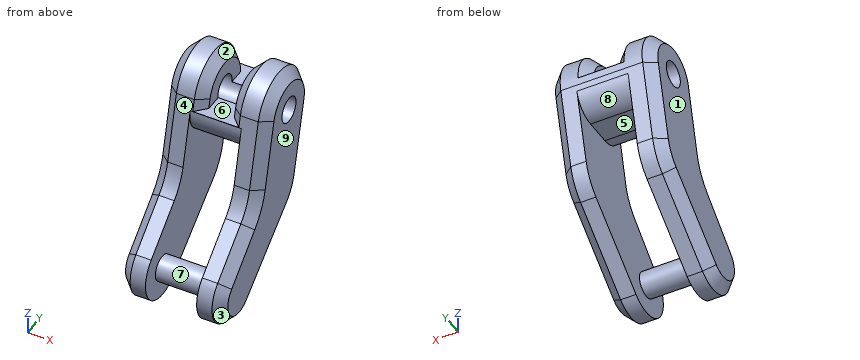
from build123d import *

# Parameters (mm, degrees)
SKETCH1_R               = 2.5
BOSS_EXTRUDE1_DEPTH     = 20
SKETCH2_W               = 10
SKETCH2_H               = 31.25301739
CUT_EXTRUDE1_DEPTH      = 26.258397403
CUT_EXTRUDE1_DEPTH_BACK = 7
FILLET1_R               = 5
CHAMFER1_SIZE           = 2
SKETCH4_R               = 2.5
BOSS_EXTRUDE2_DEPTH     = 20
SKETCH5_W               = 5
SKETCH5_H               = 8
CUT_EXTRUDE2_DEPTH      = 26.258397403
CUT_EXTRUDE2_DEPTH_BACK = 7
CHAMFER2_SIZE           = 2
SCALE1_SCALE            = 2


with BuildPart() as part:
    # Sketch1 → Boss-Extrude1 (new body)
    with BuildSketch(Plane(origin=(0, 0, 0), x_dir=(0, 0, -1), z_dir=(1, 0, 0))):
        with BuildLine():
            Line((-26.320929868, 25.036498407), (-12.043816775, 21.484201108))
            ThreePointArc((-12.043816775, 21.484201108), (-9.046440649, 20.189090541), (-6.626054873, 17.99744556))
            Line((-6.626054873, 17.99744556), (4.699352175, 3.730427474))
            ThreePointArc((4.699352175, 3.730427474), (3.853673118, -4.598826318), (-4.495069155, -3.974211028))
            Line((-4.495069155, -3.974211028), (-11.760416857, 4.243329543))
            ThreePointArc((-11.760416857, 4.243329543), (-14.097354711, 6.188634088), (-16.910883072, 7.341693702))
            Line((-16.910883072, 7.341693702), (-29.887785442, 10.466860499))
            ThreePointArc((-29.887785442, 10.466860499), (-35.416669297, 19.541837843), (-26.320929868, 25.036498407))
        make_face()
        Circle(SKETCH1_R, mode=Mode.SUBTRACT)
        with Locations((-28.13179866, 17.758397403)):
            Circle(SKETCH1_R, mode=Mode.SUBTRACT)
    extrude(amount=BOSS_EXTRUDE1_DEPTH)

    # Sketch2 → Cut-Extrude1 (cut, two sides)
    with BuildSketch(Plane(origin=(0, 0, 0), x_dir=(1, 0, 0), z_dir=(0, 1, 0))) as cut_extrude1_sk:
        with Locations((10, -5.807345092)):
            Rectangle(SKETCH2_W, SKETCH2_H)
    extrude(amount=CUT_EXTRUDE1_DEPTH, mode=Mode.SUBTRACT)
    extrude(cut_extrude1_sk.sketch, amount=-CUT_EXTRUDE1_DEPTH_BACK, mode=Mode.SUBTRACT)

    # Fillet1
    fillet1_edges = [part.edges().sort_by_distance(p)[0] for p in [
        (10, 23.820541998, 21.433853787),
        (10, 8.430939618, 21.433853787),
    ]]
    fillet(fillet1_edges, radius=FILLET1_R)

    # Chamfer1
    chamfer1_edges = [part.edges().sort_by_distance(p)[0] for p in [
        (20, 6.188634088, 14.097354711),
        (0, 8.904277101, 23.399334257),
        (0, 19.541837843, 35.416669297),
        (20, 0.134559258, 8.127743006),
        (20, -4.598826318, -3.853673118),
        (20, 10.863936517, 0.963351349),
        (20, 20.189090541, 9.046440649),
        (20, 23.260349758, 19.182373322),
        (20, 19.541837843, 35.416669297),
        (20, 8.904277101, 23.399334257),
        (0, 23.260349758, 19.182373322),
        (0, 20.189090541, 9.046440649),
        (0, 10.863936517, 0.963351349),
        (0, -4.598826318, -3.853673118),
        (0, 0.134559258, 8.127743006),
        (0, 6.188634088, 14.097354711),
    ]]
    chamfer(chamfer1_edges, length=CHAMFER1_SIZE)

    # Sketch4 → Boss-Extrude2 (add)
    with BuildSketch(Plane(origin=(20, 0, 0), x_dir=(0, 0, -1), z_dir=(1, 0, 0))):
        Circle(SKETCH4_R)
    extrude(amount=-BOSS_EXTRUDE2_DEPTH)

    # Sketch5 → Cut-Extrude2 (cut, two sides)
    with BuildSketch(Plane(origin=(0, 0, 0), x_dir=(1, 0, 0), z_dir=(0, 1, 0))) as cut_extrude2_sk:
        with Locations((10, -31.63179866)):
            Rectangle(SKETCH5_W, SKETCH5_H)
    extrude(amount=CUT_EXTRUDE2_DEPTH, mode=Mode.SUBTRACT)
    extrude(cut_extrude2_sk.sketch, amount=-CUT_EXTRUDE2_DEPTH_BACK, mode=Mode.SUBTRACT)

    # Chamfer2
    chamfer2_edges = [part.edges().sort_by_distance(p)[0] for p in [
        (7.5, 18.890459141, 35.545868812),
        (7.5, 10.195211119, 28.759792051),
        (12.5, 18.890459141, 35.545868812),
        (12.5, 10.195211119, 28.759792051),
    ]]
    chamfer(chamfer2_edges, length=CHAMFER2_SIZE)


with BuildPart() as part_1:
    # Scale1: scaled about (10, 12.009955127, 15.525619082)
    add(part.part.scale(SCALE1_SCALE).moved(Location((-10, -12.009955127, -15.525619082))))


solid = part_1.part
Source: CAD feature listing. Evaluate the final solid. Frame: model axes, mm. Face numbers are marked on the shaded views. A direction names the side the tool comes from. Coordinates: 2 decimals unless noted, no trailing zeros. Loops run counter-clockwise (first coordinate to the right, second up) from the corner with the lowest first, then second, coordinate; pieces in that order, holes last. Notation, with made-up numbers: (-12, -0.5) - (37, -0.5) arc R21 ccw to (37, 31.5) - close; hole circle Ø3 at (26, 22). An arc over 180 degrees is marked (long way). Return JSON: item names as keys, results as strings.
Q1. Mould query, pull axis X, two halves, no side actions, for the marked faces 1, 2, 3 and 4. Classes: released by +X, released by -X, zero draft, split by the parting line, or undercut.
Results:
{"face 1": "released by -X", "face 2": "undercut", "face 3": "released by +X", "face 4": "zero draft"}
Q2. Section B-B, the plane x = 9. Return loops of the section in (y, z), plus the area to 3 significant figures.
Results:
{"outline": "circle Ø10 at (-12.01, -15.53); (7.82, 39.68) arc R10 ccw to (17.55, 27.34) - (27.81, 27.34) arc R10 ccw to (37.52, 34.93) - (38.06, 37.12) arc R15 ccw to (38.47, 39.74) - (28.41, 39.74) arc R5 cw to (18.61, 39.74) - (7.84, 39.74) - close", "area": "383 mm2"}
Q3. Section A-A, the plane x = 2. Return loops of the section in (y, z).
Results:
{"outline": "circle Ø10 at (-12.01, -15.53); (7.82, 39.68) arc R10 ccw to (17.55, 27.34) - (27.81, 27.34) arc R10 ccw to (37.52, 34.93) - (38.06, 37.12) arc R15 ccw to (38.47, 39.74) - (37.47, 39.74) arc R14 ccw to (9.9, 44.02) - (8.87, 39.74) - (7.84, 39.74) - close; hole circle Ø10 at (23.51, 40.74)"}
Q4. Section C-C, the plane y = 26. Give the number of separate pieces and of enclosed holes in the cut face, plus the area to 3 significant figures.
Results:
{"separate pieces": "3", "enclosed holes": "0", "area": "1,170 mm2"}
Q5. Contact query for flat-ended pins moving along their axis: P1, Ø5, axis at x = -4, y = -5.5, coming from the +Z side; P2, Ø10, axis at y = 2, z = 27.5, coming from the -X side; P3, Ø3, axis at x = 13.5, y = 35.5, coming from the +Z side. Output: stop coordinate, or through.
Results:
{"P1": "z = 8.47", "P2": "x = -8.19", "P3": "z = 39.74"}
Q6. Section D-D, the plane z = 30. Return loops of the section in (x, y), plus the area to 3 significant figures.
Results:
{"outline": "(-10, 9.61) - (-6, 5.49) - (0, 5.49) - (0, 10.76) - (20, 10.76) - (20, 5.49) - (26, 5.49) - (30, 9.61) - (30, 32.17) - (26, 36.29) - (20, 36.29) - (20, 34.6) - (0, 34.6) - (0, 36.29) - (-6, 36.29) - (-10, 32.17) - close", "area": "1,060 mm2"}
Q7. Material intervals for line 1 along X through (y, z) = (18.5, 10); line 2 along Y through (x, z) = (-5.5, 37.5); line 3 along Z through (x, y) = (-6, 22), sorted ascending.
Results:
{"line 1": "-10 to 0, 20 to 30", "line 2": "7.3 to 19.7, 27.32 to 38.15", "line 3": "-3.85 to 35.97, 45.51 to 55.66"}
Q8. Access query for the marked faces 5, 6, 7, 8 and 9. Directions: +Z, -Z, +X, -X, +Y, -Y. A direction counts if a zero-diameter tool reaches every point of the face in a straight line with its end or side. Return the directions, or none.
Results:
{"face 5": "-Z, +Y, -Y", "face 6": "+Z, -Y", "face 7": "none", "face 8": "-Z, +Y", "face 9": "+Z, -Z, +X, +Y, -Y"}
